Build history of the part. All positions in model axes, mm. Give positions to 0.01 mm unless a question says otherwise; leave off trailing zeros. Loops run counter-clockwise (first coordinate to the right, second up) from the corner with the lowest first, then second, coordinate; pieces in that order, holes last.
1) Flat gauge pins, fed straight in: P1, Ø14.5, axis at y = 38.1, z = -342.9, coming from the -X side; P2, Ø11.5, axis at y = 38.1, z = -50.8, coming from the -X side; P3, Ø1, axis at x = 3, y = 36.5, coming from the +Z side. Where does each tip first touch, or does it go through?
2) Band-saw the part on B-B on y = 23. State how many separate pieces and enclosed holes the cut face has, then the cut area to 3 significant figures.
3) Wall check: line 1 (Y direction, x = 2, z = -196.85); line 2 (Z direction, x = 2.25, y = 38.1); line 3 (Z direction, x = 4.5, y = 78.5). Give the ranges that are in metal, low to high.
4) Band-saw the part on A-A on z = -342.9. List the corners of the cut face in (x, y), then the cut area to 3 significant figures.
Autodesk Inventor part; units mm, degrees
ref_plane "YZ Plane" through (0, 0, 0) normal (1, 0, 0) x (0, 1, 0)
ref_plane "XZ Plane" through (0, 0, 0) normal (0, 1, 0) x (-1, 0, 0)
ref_plane "XY Plane" through (0, 0, 0) normal (0, 0, 1) x (1, 0, 0)
sketch "Sketch1" plane through (0, 0, 0) normal (1, 0, 0) x (0, 1, 0)
  line L0 (444.5, 0) -> (444.5, -2.1042)
  line L1 (0, -2.1042) -> (0, 0)
  line L2 (0, -74.1174) -> (0, -66.8433)
  line L3 (0, 0) -> (82.55, 0)
  line L4 (82.55, 0) -> (82.55, -393.7)
  line L5 (82.55, -393.7) -> (0, -393.7)
  line L6 (0, -393.7) -> (0, 0)
  point P0 (25.4, -50.8)
  point P1 (25.4, -342.9)
  dimension "d2" = 82.55
  dimension "d3" = 393.7
  dimension "d4" = 50.8
  dimension "d5" = 25.4
  dimension "d6" = 50.8
  dimension "d7" = 25.4
extrude "Extrusion1" add sketch "Sketch1" along normal blind 6.35
sketch "Sketch3" plane through (6.35, 0, 0) normal (1, 0, 0) x (0, 0, -1)
  point P0 (0, 0)
sketch "Sketch4" plane through (6.35, 0, 0) normal (1, 0, 0) x (0, 0, -1)
  point P0 (0, 0)
chamfer "Chamfer1" distance 38.1 angle 45 1 edges at (3.175, 0, 0)
chamfer "Chamfer2" distance 38.1 angle 45 1 edges at (3.175, 0, -393.7)
sketch "Sketch5" plane through (0, 0, 0) normal (-1, 0, 0) x (0, 0, 1)
  line L0 (0, 82.55) -> (-393.7, 82.55)
  line L1 (-355.6, 0) -> (-393.7, 38.1)
  line L2 (-355.6, 0) -> (-38.1, 0)
  line L3 (0, 38.1) -> (-38.1, 0)
  line L4 (0, 38.1) -> (0, 82.55)
  line L5 (0, 82.55) -> (-393.7, 82.55)
  line L6 (-393.7, 82.55) -> (-393.7, 38.1)
  point P0 (0, 0)
  point P1 (-342.9, 38.1)
  point P2 (-50.8, 38.1)
  dimension "d16" = 50.8
  dimension "d17" = 38.1
  dimension "d18" = 38.1
  dimension "d19" = 50.8
hole "Hole1" at (0, 38.1, -342.9) at (0, 38.1, -50.8) direction (1, 0, 0) diameter 12.7254 end through all
sketch "Sketch7" plane through (0, 0, 0) normal (-1, 0, 0) x (0, 0, 1)
  line L0 (-38.1, 0) -> (-355.6, 0)
  line L1 (-393.7, 82.55) -> (-393.7, 38.1)
  line L2 (0, 38.1) -> (0, 82.55)
  line L3 (0, 82.55) -> (-393.7, 82.55)
  point P0 (0, 0)
  point P1 (-298.45, 10.0076)
  point P2 (-95.25, 10.0076)
  point P3 (-12.7, 78.8924)
  point P4 (-381, 78.8924)
  dimension "d42" = 10.0076
  dimension "d43" = 95.25
  dimension "d44" = 95.25
  dimension "d45" = 3.6576
  dimension "d46" = 12.7
  dimension "d47" = 12.7
  dimension "d82" = 3.6576
hole "Hole3" at (0, 78.8924, -381) at (0, 78.8924, -12.7) direction (1, 0, 0) diameter 4.7752 end through all
sketch "Sketch8" plane through (0, 0, 0) normal (-1, 0, 0) x (0, 0, 1)
  line L0 (0, 38.1) -> (0, 82.55)
  line L1 (0, 82.55) -> (-393.7, 82.55)
  line L2 (-355.6, 0) -> (-38.1, 0)
  point P0 (0, 0)
  point P1 (-196.85, 78.8924)
  point P2 (-196.85, 10.0076)
  dimension "d55" = 196.85
  dimension "d56" = 3.6576
  dimension "d57" = 10.0076
sketch "Sketch9" plane through (0, 0, 0) normal (-1, 0, 0) x (0, 0, 1)
  line L0 (-355.6, 0) -> (-38.1, 0)
  line L1 (-393.7, 82.55) -> (-393.7, 38.1)
  line L2 (0, 38.1) -> (0, 82.55)
  point P0 (0, 0)
  point P1 (-287.8836, 10.0076)
  point P2 (-105.8164, 10.0076)
  dimension "d58" = 10.0076
  dimension "d59" = 105.8164
  dimension "d60" = 105.8164
hole "Hole4" at (0, 10.0076, -196.85) direction (1, 0, 0) diameter 4.7752 end through all
hole "Hole5" at (0, 10.0076, -105.8164) at (0, 10.0076, -287.8836) direction (1, 0, 0) diameter 4.7752 end through all
sketch "Sketch10" plane through (0, 0, 0) normal (-1, 0, 0) x (0, 0, 1)
  circle A0 centre (-222.25, 36.322) radius 1.778
  circle A1 centre (-127, 36.322) radius 1.778
  line L0 (-393.7, 82.55) -> (0, 82.55)
  line L1 (-114.3619, 67.6125) -> (-112.4836, 67.6125)
  point P0 (0, 0)
  point P1 (-220.472, 36.322)
  point P2 (-128.778, 36.322)
  dimension "d108" = 46.228
  dimension "d109" = 46.228
hole "Hole6" at (0, 36.322, -127) at (0, 36.322, -220.472) at (0, 36.322, -128.778) at (0, 36.322, -222.25) direction (1, 0, 0) diameter 43.18 end through all
sketch "Sketch14" plane through (6.35, 0, 0) normal (1, 0, 0) x (0, 0, -1)
  arc A0 (127.889, 57.8937) -> (127.889, 14.7503) centre (127, 36.322) ccw
  arc A1 (127.889, 14.7503) -> (127.889, 57.8937) centre (128.778, 36.322) ccw
  arc A2 (221.361, 57.8937) -> (221.361, 14.7503) centre (220.472, 36.322) ccw
  arc A3 (221.361, 14.7503) -> (221.361, 57.8937) centre (222.25, 36.322) ccw
  line L0 (127.889, 57.8937) -> (127.889, 14.7503)
  line L1 (96.03, 36.322) -> (156.5626, 36.322)
  line L2 (221.361, 57.8937) -> (221.361, 14.7503)
  line L3 (190.5646, 36.322) -> (248.6345, 36.322)
  line L4 (127.889, 36.322) -> (103.886, 36.322)
  line L5 (103.886, 36.322) -> (103.886, 43.3324)
  line L6 (103.886, 43.3324) -> (103.886, 36.322)
  line L7 (103.886, 36.322) -> (103.886, 29.3116)
  line L8 (127.889, 36.322) -> (151.892, 36.322)
  line L9 (151.892, 36.322) -> (151.892, 29.3116)
  line L10 (151.892, 36.322) -> (151.892, 43.3324)
  line L11 (221.361, 43.3324) -> (197.358, 43.3324)
  line L12 (221.361, 43.3324) -> (245.364, 43.3324)
  line L13 (221.361, 29.3116) -> (197.358, 29.3116)
  line L14 (221.361, 29.3116) -> (245.364, 29.3116)
  circle A4 centre (103.886, 29.3116) radius 1.7526
  circle A5 centre (103.886, 43.3324) radius 1.7526
  circle A6 centre (151.892, 43.3324) radius 1.7526
  circle A7 centre (151.892, 29.3116) radius 1.7526
  circle A8 centre (197.358, 43.3324) radius 1.7526
  circle A9 centre (197.358, 29.3116) radius 1.7526
  circle A10 centre (245.364, 29.3116) radius 1.7526
  circle A11 centre (245.364, 43.3324) radius 1.7526
  point P0 (0, 0)
  dimension "d113" = 24.003
  dimension "d114" = 7.0104
  dimension "d115" = 7.0104
  dimension "d116" = 24.003
  dimension "d117" = 24.003
  dimension "d118" = 24.003
  dimension "d119" = 3.5052
  dimension "d120" = 3.5052
  dimension "d121" = 3.5052
  dimension "d122" = 3.5052
  dimension "d123" = 3.5052
extrude "Extrusion2" cut sketch "Sketch14" against normal blind 25.4 contours A6 | A7 | A4 | A5 | A11 | A10 | A9 | A8
properties part number "DriveTrainPlate"
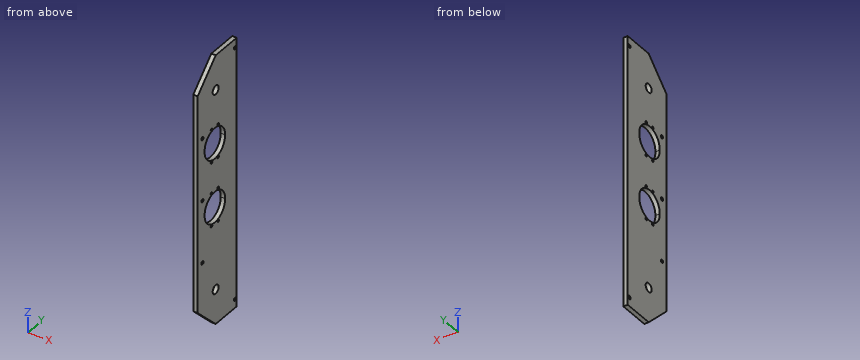
Findings below:
1. P1: stops at x = 0
1. P2: passes through
1. P3: stops at z = -1.1
2. separate pieces: 3
2. enclosed holes: 0
2. area: 1,850 mm2
3. line 1: y = 0 to 7.62, 12.4 to 27.63, 30.99 to 41.66, 45.01 to 82.55
3. line 2: z = -393.7 to -349.26, -336.54 to -243.77, -198.96 to -150.29, -105.48 to -57.16, -44.44 to 0
3. line 3: z = -393.7 to -383.36, -378.64 to -15.06, -10.34 to 0
4. outline: (0, 0) - (6.35, 0) - (6.35, 31.74) - (0, 31.74) - close; (0, 44.46) - (6.35, 44.46) - (6.35, 82.55) - (0, 82.55) - close
4. area: 443 mm2
